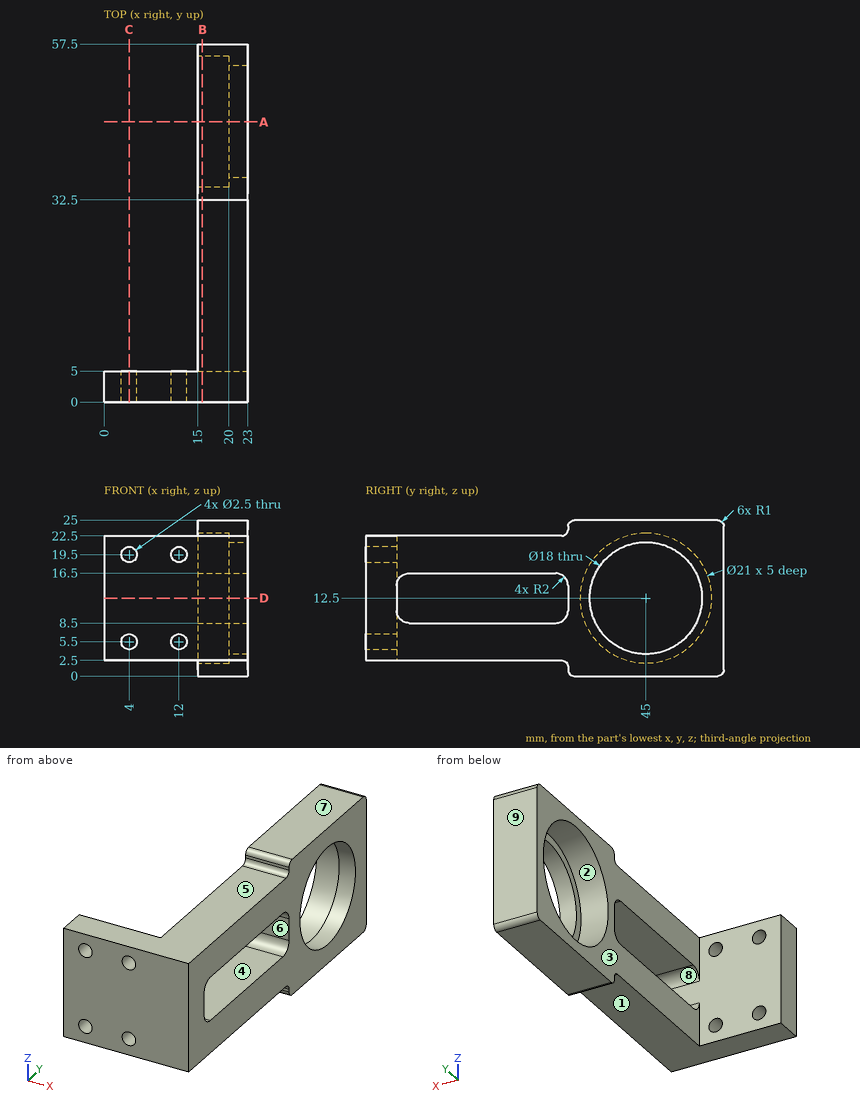
Drawing for the job (mm, zero at the part's lowest x, y, z). A direction names the side the tool comes from. Give positions to 0.01 mm unless a question says otherwise; leave off trailing zeros. Write each loop counter-clockwise with the first axis right and the second up, starting at its lowest first coordinate (ties: lowest second). Pieces come first, ordered by that corner, then holes. Notation, with made-up numbers: M 14,81.5 L 45,81.5 A22 ccw 45,90.5 Z; hole C 89,-5.75 d8. An arc over 180 degrees is marked long. Use CSV: the item, a comma, the result in double quotes.
Item 1: Slice it at C-C on x = 4. Write the cut outline in (y, z), plus the area to 3 significant figures.
Taken from the geometry:
outline,"M 0,2.5 L 5,2.5 L 5,4.25 L 0,4.25 Z; M 0,6.75 L 5,6.75 L 5,18.25 L 0,18.25 Z; M 0,20.75 L 5,20.75 L 5,22.5 L 0,22.5 Z"
area,"75.0 mm²"
Item 2: Drill centre lines: probe 1 along X at (y, z) = (1.75, 5.5); probe 2 along Y at (x, z) = (19.75, 10); probe 3 along Z at (x, y) = (21.25, 16). Where is each one in solid material? Low to high.
Taken from the geometry:
probe 1,"x = 0 to 2.75, 5.25 to 10.75, 13.25 to 23"
probe 2,"y = 0 to 5.06, 32.44 to 34.8, 55.2 to 57.5"
probe 3,"z = 2.5 to 8.5, 16.5 to 22.5"
Item 3: Slice it at A-A on y = 45. Write the cut outline in (x, z).
Taken from the geometry:
outline,"M 15,0 L 23,0 L 23,3.5 L 20,3.5 L 20,2 L 15,2 Z; M 15,23 L 20,23 L 20,21.5 L 23,21.5 L 23,25 L 15,25 Z"
Item 4: Which spindle directions (+Z, -Z, +X, -X, +Y, -Y) get a long thin tool onto all of the face, cutting with end or side? Do the marked faces 1, 2, 3, 4 and 5. Say none if no direction does.
Taken from the geometry:
face 1,"-Z, +X, -X, -Y"
face 2,"-X"
face 3,"+Z, -Z, -X, +Y"
face 4,"+X, -X"
face 5,"+Z, +X, -X, -Y"
Item 5: Slice it at D-D on z = 12.5. Write the cut outline in (x, y).
Taken from the geometry:
outline,"M 0,0 L 23,0 L 23,5 L 0,5 Z; M 15,32.5 L 23,32.5 L 23,36 L 20,36 L 20,34.5 L 15,34.5 Z; M 15,55.5 L 20,55.5 L 20,54 L 23,54 L 23,57.5 L 15,57.5 Z"
Item 6: Slice it at B-B on x = 15.75. Write the cut outline in (y, z).
Taken from the geometry:
outline,"M 0,2.5 L 31.5,2.5 A1 cw 32.5,1.5 L 32.5,1 A1 ccw 33.5,0 L 56.5,0 A1 ccw 57.5,1 L 57.5,24 A1 ccw 56.5,25 L 33.5,25 A1 ccw 32.5,24 L 32.5,23.5 A1 cw 31.5,22.5 L 0,22.5 Z; hole M 5,10.5 A2 ccw 7,8.5 L 30.5,8.5 A2 ccw 32.5,10.5 L 32.5,14.5 A2 ccw 30.5,16.5 L 7,16.5 A2 ccw 5,14.5 Z; hole C 45,12.5 d21"
Item 7: Pull direction Z, two halves, no side cores. Call the marked faces 6, 7, 8 and 9: +Z half, -Z half, draft (parallel to the pull), parting line (faces both ways), or undercut.
Taken from the geometry:
face 6,"undercut"
face 7,"+Z half"
face 8,"undercut"
face 9,"draft"
Item 8: Pin check, flat tips, straight feed: P1, Ø8, axis at y = 44, z = 9, coming from the -X side; P2, Ø6.5, axis at x = 19, y = 15.5, coming from the -Z side; P3, Ø7.5, axis at y = 29.5, z = 8, coming from the -X side; P4, Ø0.6, axis at x = 17.5, z = 23.5, coming from the -Y side. Stop position of each tip, or through.
Taken from the geometry:
P1,"passes through"
P2,"stops at z = 2.5"
P3,"stops at x = 15"
P4,"stops at y = 32.45"
